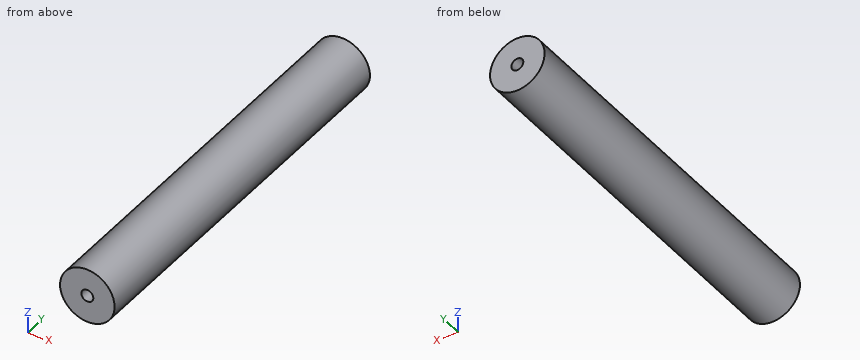
```python
from build123d import *

# Parameters (mm, degrees)
SKETCH_1_R      = 7.5
EXTRUDE_1_DEPTH = 105


with BuildPart() as part:
    # ｽｹｯﾁ1 → ﾎﾞｽ - 押し出し1 (new body)
    with BuildSketch(Plane(origin=(0, 0, 0), x_dir=(1, 0, 0), z_dir=(0, 1, 0))):
        with Locations(Location((0, 0, 0), (0, 0, 270))):
            Circle(SKETCH_1_R)
    extrude(amount=EXTRUDE_1_DEPTH)

    # ｽｹｯﾁ3 → M4x0.7 ねじ穴1 (revolve, cut)
    with BuildSketch(Plane(origin=(0, 105, 0), x_dir=(0, 0, 1), z_dir=(1, 0, 0))):
        Polygon((0, 0), (0, 20.991420021), (1.65, 20), (1.65, 0), align=None)
    m4x0_7_1 = revolve(axis=Axis((0, 111.35, 0), (0, -1, 0)), mode=Mode.SUBTRACT)

    # ﾐﾗｰ1: M4x0.7 ねじ穴1 across plane
    add(m4x0_7_1.mirror(Plane.ZX.offset(52.5)), mode=Mode.SUBTRACT)


solid = part.part
```
Work out the finished part from the listing and answer in its coordinate system (mm). Round coordinates to 2 decimals unless told otherwise and drop trailing zeros. Write each loop counter-clockwise with the first axis right and the second up, starting at its lowest first coordinate (ties: lowest second). Pieces come first, ordered by that corner, then holes. Notation, with made-up numbers: (-38, 27.5) -> (-10, 27.5) arc R25 ccw to (-10, 44.5) -> close; hole circle Ø3 at (87.5, -22). An arc over 180 degrees is marked (long way). Write each question's results on one line, items separated by ' | '.
1) Consider line 1 along X through (y, z) = (95, 0); line 2 along Z through (x, y) = (1.5, 90); line 3 along Z through (x, y) = (-3, 55). Determine where each line is inside the solid, lowest interval first. Write a range as [from, to].
Findings:
line 1: x = [-7.5, -1.65], [1.65, 7.5] | line 2: z = [-7.35, -0.69], [0.69, 7.35] | line 3: z = [-6.87, 6.87]
2) The part is cut by section C-C (z = 5.25). Write down the section's boundary in (x, y).
Findings:
outline: (-5.36, 0) -> (5.36, 0) -> (5.36, 105) -> (-5.36, 105) -> close
3) The part is cut by section A-A (y = 97). Write down the section's boundary in (x, z), and give its area (3 significant figures).
Findings:
outline: circle Ø15 at (0, 0); hole circle Ø3.3 at (0, 0) | area: 168 mm²
4) The part is cut by section D-D (x = 5.25). Write down the section's boundary in (y, z).
Findings:
outline: (0, -5.36) -> (105, -5.36) -> (105, 5.36) -> (0, 5.36) -> close
5) The part is cut by section B-B (y = 27.5). Write down the section's boundary in (x, z).
Findings:
outline: circle Ø15 at (0, 0)
6) Flat-ended cylindrical pins translate along their axes: pin 1 (2 mm diameter, centred on x = -4.5, z = -1.5, fed in from -Y); pin 2 (2 mm diameter, centred on x = 3, y = 78, fed in from -Z); pin 3 (1 mm diameter, centred on y = 64, z = -4, fed in from +X); pin 4 (2.5 mm diameter, centred on x = 0, z = 0, fed in from +Y). Find the tip coordinate at first contact, or state that the pin passes through.
Findings:
pin 1: stops at y = 0 | pin 2: stops at z = -7.23 | pin 3: stops at x = 6.63 | pin 4: stops at y = 84.76
